Design review of the part built by this model. Coordinates are the model's own, in mm. A direction names the side the tool comes from. Give positions to 0.01 mm unless a question says otherwise; leave off trailing zeros. Loops run counter-clockwise (first coordinate to the right, second up) from the corner with the lowest first, then second, coordinate; pieces in that order, holes last. Notation, with made-up numbers: (52, -22.75) -> (82, -22.75) arc R17 cw to (82, -9.75) -> close; hole circle Ø6 at (-18, -35). An arc over 180 degrees is marked (long way). Answer in a Markdown table with one row per item. Add a question column.
(1) Consider section B-B on y = 1.65. Count the separate pieces of the cut face and the enclosed holes in it, then the cut area to 3 significant figures.
(2) Consider section D-D on x = -125.5. Write out the cut boundary in (y, z), then the cut area to 3 significant figures.
(3) Consider section A-A on z = 32. Write out the cut boundary in (x, y), then the cut area to 3 significant figures.
(4) Draft analysis for pull direction X (two halves, no side actions). For faces 3 (the flat face through (-112.985, 1.479, 64.113)), 4 (the flat face through (112.985, 1.479, -64.113)), 5 (the cylindrical face through (-4.274, 1.521, 44.671)), state which applies: +X half, -X half, draft (parallel to the pull), parting line (faces both ways), or undercut.
(5) Consider section C-C on z = -91.5. Write out the cut boundary in (x, y), then the cut area to 3 significant figures.
(6) For faces 1 (the flat face through (-2, 3, -2)), 2 (the flat face through (15.975, 1.521, -27.08)), list the 3-axis set-ups (+Z, -Z, +X, -X, +Y, -Y) from which the entire face can be reached by the end or side of a thin tool; tool diameter is ignored.
(7) For pin 1 (2.5 mm diameter, centred on x = 59.63, z = 16.53, fed in from +Y), flat-tipped, find the tip position at first contact; note if it passes through.
(8) For line 1 (Z direction, x = 103, y = 2.4); line 2 (X direction, y = 1.6, z = 1); line 3 (Z direction, x = 89, y = 0.75), list the stretches that pass through material, from the lowest coordinate up.
from build123d import *

# Parameters (mm, degrees)
ESQUISSE1_R             = 2
BOSS_EXTRU_1_DEPTH      = 3
CONG_2_R                = 10
CONG_3_R                = 10
ENL_V_MAT_EXTRU_1_DEPTH = 198.287332615


with BuildPart() as part:
    # Esquisse1 → Boss.-Extru.1 (new body)
    with BuildSketch(Plane(origin=(0, 0, 0), x_dir=(1, 0, 0), z_dir=(0, 1, 0))):
        Polygon((-150, 0), (-75, -129.903810568), (75, -129.903810568), (150, 0), (75, 129.903810568), (-75, 129.903810568), align=None)
        with Locations(Location((15.5, -109.903810568, 0), (0, 0, 270))):
            Circle(ESQUISSE1_R, mode=Mode.SUBTRACT)
        with Locations(Location((-15.5, -109.903810568, 0), (0, 0, 90))):
            Circle(ESQUISSE1_R, mode=Mode.SUBTRACT)
        with Locations(Location((15.5, -59.903810568, 0), (0, 0, 270))):
            Circle(ESQUISSE1_R, mode=Mode.SUBTRACT)
        with Locations(Location((-15.5, -59.903810568, 0), (0, 0, 90))):
            Circle(ESQUISSE1_R, mode=Mode.SUBTRACT)
        with Locations(Location((-87.429491924, -68.375299042, 0), (0, 0, 270))):
            Circle(ESQUISSE1_R, mode=Mode.SUBTRACT)
        with Locations(Location((-102.929491924, -41.528511525, 0), (0, 0, 90))):
            Circle(ESQUISSE1_R, mode=Mode.SUBTRACT)
        with Locations(Location((-59.628221735, -16.528511525, 0), (0, 0, 90))):
            Circle(ESQUISSE1_R, mode=Mode.SUBTRACT)
        with Locations(Location((-44.128221735, -43.375299042, 0), (0, 0, 270))):
            Circle(ESQUISSE1_R, mode=Mode.SUBTRACT)
        with Locations(Location((-102.929491924, 41.528511525, 0), (0, 0, 270))):
            Circle(ESQUISSE1_R, mode=Mode.SUBTRACT)
        with Locations(Location((-87.429491924, 68.375299042, 0), (0, 0, 90))):
            Circle(ESQUISSE1_R, mode=Mode.SUBTRACT)
        with Locations(Location((-44.128221735, 43.375299042, 0), (0, 0, 90))):
            Circle(ESQUISSE1_R, mode=Mode.SUBTRACT)
        with Locations(Location((-59.628221735, 16.528511525, 0), (0, 0, 270))):
            Circle(ESQUISSE1_R, mode=Mode.SUBTRACT)
        with Locations(Location((-15.5, 109.903810568, 0), (0, 0, 270))):
            Circle(ESQUISSE1_R, mode=Mode.SUBTRACT)
        with Locations(Location((15.5, 109.903810568, 0), (0, 0, 90))):
            Circle(ESQUISSE1_R, mode=Mode.SUBTRACT)
        with Locations(Location((15.5, 59.903810568, 0), (0, 0, 90))):
            Circle(ESQUISSE1_R, mode=Mode.SUBTRACT)
        with Locations(Location((-15.5, 59.903810568, 0), (0, 0, 270))):
            Circle(ESQUISSE1_R, mode=Mode.SUBTRACT)
        with Locations(Location((87.429491924, 68.375299042, 0), (0, 0, 270))):
            Circle(ESQUISSE1_R, mode=Mode.SUBTRACT)
        with Locations(Location((102.929491924, 41.528511525, 0), (0, 0, 90))):
            Circle(ESQUISSE1_R, mode=Mode.SUBTRACT)
        with Locations(Location((59.628221735, 16.528511525, 0), (0, 0, 90))):
            Circle(ESQUISSE1_R, mode=Mode.SUBTRACT)
        with Locations(Location((44.128221735, 43.375299042, 0), (0, 0, 270))):
            Circle(ESQUISSE1_R, mode=Mode.SUBTRACT)
        with Locations(Location((102.929491924, -41.528511525, 0), (0, 0, 270))):
            Circle(ESQUISSE1_R, mode=Mode.SUBTRACT)
        with Locations(Location((87.429491924, -68.375299042, 0), (0, 0, 90))):
            Circle(ESQUISSE1_R, mode=Mode.SUBTRACT)
        with Locations(Location((44.128221735, -43.375299042, 0), (0, 0, 90))):
            Circle(ESQUISSE1_R, mode=Mode.SUBTRACT)
        with Locations(Location((59.628221735, -16.528511525, 0), (0, 0, 270))):
            Circle(ESQUISSE1_R, mode=Mode.SUBTRACT)
    extrude(amount=BOSS_EXTRU_1_DEPTH)

    # Congé2
    cong_2_edges = [part.edges().sort_by_distance(p)[0] for p in [
        (-75, 1.5, -129.903810568),
    ]]
    fillet(cong_2_edges, radius=CONG_2_R)

    # Congé3
    cong_3_edges = [part.edges().sort_by_distance(p)[0] for p in [
        (75, 1.5, -129.903810568),
        (150, 1.5, 0),
        (75, 1.5, 129.903810568),
        (-75, 1.5, 129.903810568),
        (-150, 1.5, 0),
    ]]
    fillet(cong_3_edges, radius=CONG_3_R)

    # Esquisse3 → Enlèv. mat.-Extru.1 (cut, through all)
    with BuildSketch(Plane(origin=(0, 3, 0), x_dir=(1, 0, 0), z_dir=(0, 1, 0))):
        with BuildLine():
            Line((2.5, 46.406387956), (38.939110868, 25.368257487))
            ThreePointArc((38.939110868, 25.368257487), (40.769237886, 18.538130468), (33.939110868, 16.708003449))
            Line((33.939110868, 16.708003449), (-2.5, 37.746133918))
            ThreePointArc((-2.5, 37.746133918), (-4.330127019, 44.576260937), (2.5, 46.406387956))
        make_face()
        with BuildLine():
            Line((38.939110868, -25.368257487), (2.5, -46.406387956))
            ThreePointArc((2.5, -46.406387956), (-4.330127019, -44.576260937), (-2.5, -37.746133918))
            Line((-2.5, -37.746133918), (33.939110868, -16.708003449))
            ThreePointArc((33.939110868, -16.708003449), (40.769237886, -18.538130468), (38.939110868, -25.368257487))
        make_face()
        with BuildLine():
            Line((-41.439110868, -21.038130468), (-41.439110868, 21.038130468))
            ThreePointArc((-41.439110868, 21.038130468), (-36.439110868, 26.038130468), (-31.439110868, 21.038130468))
            Line((-31.439110868, 21.038130468), (-31.439110868, -21.038130468))
            ThreePointArc((-31.439110868, -21.038130468), (-36.439110868, -26.038130468), (-41.439110868, -21.038130468))
        make_face()
    extrude(amount=-ENL_V_MAT_EXTRU_1_DEPTH, mode=Mode.SUBTRACT)


solid = part.part
Values follow:
| question | item | result |
|---|---|---|
| 1 | separate pieces | 1 |
| 1 | enclosed holes | 27 |
| 1 | area | 56,600 mm2 |
| 2 | outline | (0, -42.44) -> (3, -42.44) -> (3, 42.44) -> (0, 42.44) -> close |
| 2 | area | 255 mm2 |
| 3 | outline | (-131.52, 0) -> (7.45, 0) -> (7.45, 3) -> (-131.52, 3) -> close; (27.45, 0) -> (131.52, 0) -> (131.52, 3) -> (27.45, 3) -> close |
| 3 | area | 729 mm2 |
| 4 | face 3 | -X half |
| 4 | face 4 | +X half |
| 4 | face 5 | undercut |
| 5 | outline | (-97.17, 0) -> (97.17, 0) -> (97.17, 3) -> (-97.17, 3) -> close |
| 5 | area | 583 mm2 |
| 6 | face 1 | +Z, -Z, +X, -X, +Y |
| 6 | face 2 | +Y, -Y |
| 7 | pin 1 | through |
| 8 | line 1 | -81.41 to -43.53, -39.53 to 39.53, 43.53 to 81.41 |
| 8 | line 2 | -148.4 to -41.44, -31.44 to 148.4 |
| 8 | line 3 | -105.66 to -69.61, -67.14 to 67.14, 69.61 to 105.66 |
